Autodesk Inventor part; units mm, degrees
ref_plane "YZ Plane" through (0, 0, 0) normal (1, 0, 0) x (0, 1, 0)
ref_plane "XZ Plane" through (0, 0, 0) normal (0, 1, 0) x (-1, 0, 0)
ref_plane "XY Plane" through (0, 0, 0) normal (0, 0, 1) x (1, 0, 0)
sketch "Sketch1" plane through (0, 0, 0) normal (0, 1, 0) x (-1, 0, 0)
  line L0 (-26.2289, 0) -> (-26.2289, -40)
  line L1 (-0.4496, -40) -> (-0.4496, 0)
  circle A0 centre (-33.2736, -30) radius 1.55
  circle A1 centre (6.595, -30) radius 1.55
  circle A2 centre (-33.2736, -10) radius 1.55
  circle A3 centre (6.595, -10) radius 1.55
  circle A4 centre (-15.5193, -10) radius 6.4
  circle A5 centre (-23.0443, -37.6) radius 1.05
  circle A6 centre (-7.9943, -37.6) radius 1.05
  circle A7 centre (-23.0443, -22.5) radius 1.05
  circle A8 centre (-7.9943, -22.5) radius 1.05
  circle A9 centre (-23.0443, -2.5) radius 1.05
  circle A10 centre (-7.9943, -2.5) radius 1.05
  arc A11 (13.19, -1) -> (12.19, 0) centre (12.19, -1) ccw
  line L2 (-38.8686, 0) -> (12.19, 0)
  arc A12 (-38.8686, 0) -> (-39.8686, -1) centre (-38.8686, -1) ccw
  line L3 (-39.8686, -39) -> (-39.8686, -1)
  arc A13 (-39.8686, -39) -> (-38.8686, -40) centre (-38.8686, -39) ccw
  arc A14 (12.19, -40) -> (13.19, -39) centre (12.19, -39) ccw
  line L4 (12.19, -40) -> (-38.8686, -40)
  line L5 (13.19, -1) -> (13.19, -39)
  line L6 (-26.6786, -40) -> (-26.6786, 0)
  line L7 (-25.7793, 0) -> (-25.7793, -40)
  line L8 (-0.8993, -40) -> (-0.8993, 0)
  line L9 (0, 0) -> (0, -40)
  point P0 (0, 0)
extrude "Extrusion1" add sketch "Sketch1" against normal blind 1.5
properties part number "body_motor_R_frame"
Geometry check sheet. Reference: the model listing, model coordinates, mm. Round coordinates to 2 decimals unless told otherwise and drop trailing zeros. Order: outer loops, then holes, each group sorted by start corner. A loop starts at its lowest first (then second) coordinate and runs counter-clockwise, first axis right, second up. Notation, with made-up numbers: M 26.5,48 L 44.5,48 A25 ccw 44.5,87 Z; hole C 26.25,13 d7. An arc over 180 degrees is marked long. Answer in a Markdown table with one row per item. Add a question column.
Item 1: Depth check by flat-ended pin: pin 1 Ø1.7 at (x, z) = (23.04, -2.5) entering from -Y. Enter the tip coordinate at first touch or a pass-through.
Item 2: Sectioned sample at B-B, the plane y = -0.9. State how many separate pieces and enclosed holes the cut face has, plus the area to 3 significant figures.
Item 3: Draft check along X on faces 1 (the face through (13, -1, -40)), 2 (the face through (-12.905, -0.74, -0.301)), 3 (the face through (33.475, -0.74, -28.463)). Enter one of: released by +X, released by -X, zero draft, split by the parting line, or undercut.
Item 4: Material ranges on L1, parallel to X at y = -0.85, z = -2; L2, parallel to Z at x = -7, y = -0.4; L3, parallel to Z at x = 23.5, y = -0.5, recorded low to high. Write a range as [from, to].
Item 5: Sectioned sample at C-C, the plane z = -5.5. Enter the section's corners in (x, y), plus the area to 3 significant figures.
Item 6: Sectioned sample at A-A, the plane z = -22.5. Enter the section's corners in (x, y).
Item 7: Sectioned sample at D-D, the plane z = -30. Enter the section's corners in (x, y) (3 decimals).
Filled in:
| question | item | result |
|---|---|---|
| 1 | pin 1 | passes through |
| 2 | separate pieces | 1 |
| 2 | enclosed holes | 11 |
| 2 | area | 1,940 mm² |
| 3 | face 1 | zero draft |
| 3 | face 2 | released by -X |
| 3 | face 3 | undercut |
| 4 | L1 | x = [-13.19, 7.07], [8.92, 22.12], [23.97, 39.87] |
| 4 | L2 | z = [-40, -31.5], [-28.5, -11.5], [-8.5, 0] |
| 4 | L3 | z = [-40, -38.55], [-36.65, -23.45], [-21.55, -3.45], [-1.55, 0] |
| 5 | outline | M -13.19,-1.5 L 10.97,-1.5 L 10.97,0 L -13.19,0 Z; M 20.07,-1.5 L 39.87,-1.5 L 39.87,0 L 20.07,0 Z |
| 5 | area | 65.9 mm² |
| 6 | outline | M -13.19,-1.5 L 6.94,-1.5 L 6.94,0 L -13.19,0 Z; M 9.04,-1.5 L 21.99,-1.5 L 21.99,0 L 9.04,0 Z; M 24.09,-1.5 L 39.87,-1.5 L 39.87,0 L 24.09,0 Z |
| 7 | outline | M -13.19,-1.5 L -8.145,-1.5 L -8.145,0 L -13.19,0 Z; M -5.045,-1.5 L 31.724,-1.5 L 31.724,0 L -5.045,0 Z; M 34.824,-1.5 L 39.869,-1.5 L 39.869,0 L 34.824,0 Z |
